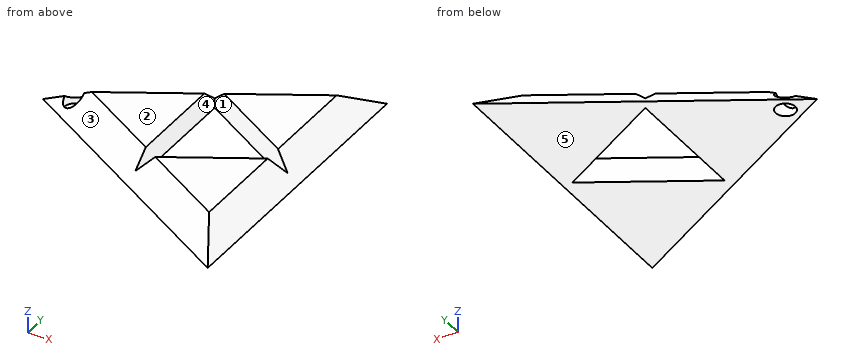
```python
from build123d import *

# Parameters (mm, degrees)
F1_DEPTH    = 5
F2_R        = 2
F3_DEPTH    = 25
F4_T1_DEPTH = 85.7168298797
F4_T3_DEPTH = 85.7168298797
F4_T5_DEPTH = 85.7168298797


# Not quite as in the source:
# - a fillet or chamfer that OpenCascade refuses, or shapes differently, is made with other operations: its cross-section is extruded or revolved along the edge and cut away or added


with BuildPart() as f1:
    # F0 (on Top) → F1 (new body)
    with BuildSketch(Plane.XY):
        Polygon((17.3205080757, -30), (17.3205080757, 30), (-34.6410161514, 0), align=None)
        Polygon((-7.6602540378, -13.2679491924), (-7.6602540378, 13.2679491924), (15.3205080757, 0), align=None, mode=Mode.SUBTRACT)
    extrude(amount=F1_DEPTH)

    # F2 (on face) → F3 (cut)
    with BuildSketch(Plane.XY.offset(5)):
        with Locations((-28.2111279666, 0)):
            Circle(F2_R)
    extrude(amount=-F3_DEPTH, mode=Mode.SUBTRACT)

    # F4: chamfer of 5 on 3 edges, made by hand

    # F4_s2 → F4_t1 (cut)
    with BuildSketch(Plane(origin=(37.1164761038, 21.4292074699, 0), x_dir=(0, 0, 1), z_dir=(-0.8660254038, -0.5, 0))):
        Polygon((0, 17.3205080757), (5, 12.3205080757), (5, 17.3205080757), align=None)
    extrude(amount=F4_T1_DEPTH, mode=Mode.SUBTRACT)

    # F4_s4 → F4_t3 (cut)
    with BuildSketch(Plane.XZ.offset(-42.8584149398)):
        Polygon((17.3205080757, 0), (12.3205080757, 5), (17.3205080757, 5), align=None)
    extrude(amount=F4_T3_DEPTH, mode=Mode.SUBTRACT)

    # F4_s6 → F4_t5 (cut)
    with BuildSketch(Plane(origin=(-37.1164761038, 21.4292074699, 0), x_dir=(0, 0, 1), z_dir=(0.8660254038, -0.5, 0))):
        Polygon((0, 17.3205080757), (5, 12.3205080757), (5, 17.3205080757), align=None)
    extrude(amount=F4_T5_DEPTH, mode=Mode.SUBTRACT)


solid = f1.part
```
Verification items for the finished model (mm, model axes). Face numbers are marked on the shaded views. A direction names the side the tool comes from. Give positions to 0.01 mm unless a question says otherwise; leave off trailing zeros. Order: outer loops, then holes, each group sorted by start corner. A loop starts at its lowest first (then second) coordinate and runs counter-clockwise, first axis right, second up. Notation, with made-up numbers: (21.25, 42.5) - (65.25, 42.5) arc R14 cw to (65.25, 67.5) - close; hole circle Ø4 at (74.5, 51.25). An arc over 180 degrees is marked (long way). Answer as CSV lines item,"result". Start each with the question number.
Item 1: Gauge pin test, flat ends, axial feed: pin 1 (8 mm diameter, centred on x = -18.5, y = 13.5, fed in from +Z); pin 2 (6 mm diameter, centred on x = 1, y = -23, fed in from -Z). Record the tip position at first contact, or that the pin passes through.
Item 2: Section check D-D, the plane x = 13.5. Record the boundary of the cut face in (y, z).
Item 3: Section check C-C, the plane y = 6. Record the boundary of the cut face in (x, z), plus the area to 3 significant figures.
Item 4: Section check A-A, the plane x = -27.5. Record the boundary of the cut face in (y, z).
Item 5: Access from +Z, -Z, +X, -X, +Y, -Y to the whole of each face (thin tool, end or side, straight path). Record for the marked faces 4 and 5.
Item 6: Material ranges on L1, parallel to X at y = 0, z = 2.5; L2, parallel to Y at x = -1.5, z = 1.9; L3, parallel to X at y = -6, z = 3.8, recorded low to high.
Item 7: Mould release check, pull along Y, two halves, no side actions. Record for the marked faces 1, 2 and 3: released by +Y, released by -Y, zero draft, split by the parting line, or undercut.
Item 8: Section check B-B, the plane z = 3.25. Record the boundary of the cut face in (x, y).
Filled in:
1,pin 1,"z = 0.38"
1,pin 2,"z = 0"
2,outline,"(-27.79, 0) - (-1.05, 0) - (-1.05, 3.82) - (-23.38, 3.82) - close; (1.05, 0) - (27.79, 0) - (23.38, 3.82) - (1.05, 3.82) - close"
3,outline,"(-24.25, 0) - (-7.66, 0) - (-7.66, 5) - (-14.25, 5) - close; (4.93, 0) - (17.32, 0) - (12.32, 5) - (4.93, 5) - close"
3,area,"107 mm^2"
4,outline,"(-4.12, 0) - (-1.87, 0) - (-1.87, 1.95) - close; (1.87, 0) - (4.12, 0) - (1.87, 1.95) - close"
5,face 4,"+Z, -Z"
5,face 5,"-Z, +X, -X, +Y, -Y"
6,L1,"-26.21 to -7.66"
6,L2,"-16.94 to -9.71, 9.71 to 16.94"
6,L3,"-16.65 to -7.66, 4.93 to 13.52"
7,face 1,"undercut"
7,face 2,"zero draft"
7,face 3,"released by -Y"
8,outline,"(-26.46, -0.97) - (-7.66, -11.82) - (-7.66, 11.82) - (-26.46, 0.97) arc R2 cw to start; (-6.41, -12.55) - (14.07, -24.37) - (14.07, -0.72) - close; (-6.41, 12.55) - (14.07, 0.72) - (14.07, 24.37) - close"
